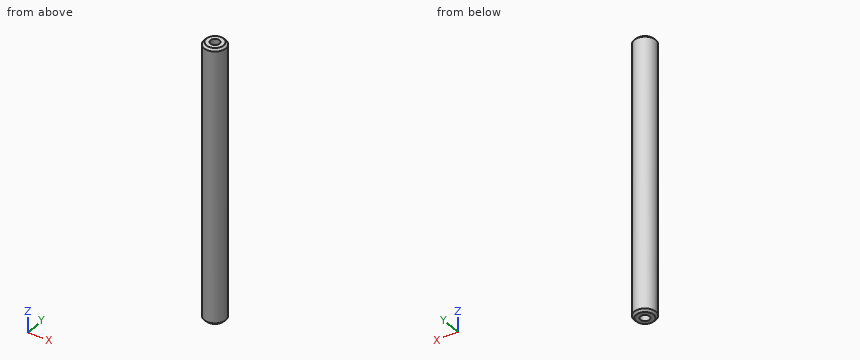
```python
from build123d import *

# Parameters (mm, degrees)
SKETCH3_R           = 3.96875
BOSS_EXTRUDE1_DEPTH = 50.8
CHAMFER1_SIZE       = 0.79375


with BuildPart() as part:
    # Sketch3 → Boss-Extrude1 (new body, symmetric)
    with BuildSketch(Plane.XY):
        Circle(SKETCH3_R)
    extrude(amount=BOSS_EXTRUDE1_DEPTH, both=True)

    # Chamfer1
    chamfer1_edges = [part.edges().sort_by_distance(p)[0] for p in [
        (-3.96875, 0, -50.8),
        (-3.96875, 0, 50.8),
    ]]
    chamfer(chamfer1_edges, length=CHAMFER1_SIZE)

    # Sketch6 → M4x0.7 Tapped Hole1 (revolve, cut)
    with BuildSketch(Plane(origin=(0, 0, -50.8), x_dir=(0, 1, 0), z_dir=(1, 0, 0))):
        Polygon((0, 0), (0, 15.991420021), (1.65, 15), (1.65, 0), align=None)
    m4x0_7_tapped_hole1 = revolve(axis=Axis((0, 0, -57.15), (0, 0, 1)), mode=Mode.SUBTRACT)

    # Mirror1: M4x0.7 Tapped Hole1 across plane
    add(m4x0_7_tapped_hole1.mirror(Plane.XY), mode=Mode.SUBTRACT)


solid = part.part
```
The model under review builds one solid part; all positions refer to its coordinate system, in mm. Round coordinates to 2 decimals unless told otherwise and drop trailing zeros. Order: outer loops, then holes, each group sorted by start corner. A loop starts at its lowest first (then second) coordinate and runs counter-clockwise, first axis right, second up. Notation, with made-up numbers: M 85,-26 L 123,-26 A22 ccw 123,-16 Z; hole C -30,53.5 d11. An arc over 180 degrees is marked long. Use a Markdown table: item, result.
1) Insertion check: pin 1 (2 mm diameter, centred on x = 1.5, z = -25, fed in from -Y); pin 2 (3 mm diameter, centred on x = 0, y = 0, fed in from -Z); pin 3 (1.5 mm diameter, centred on y = 3, z = 31.5, fed in from -X). Each pin has a flat end and moves straight along its axis. Give the tip position at first contact, or say it passes through.
Report:
| item | result |
|---|---|
| pin 1 | y = -3.94 |
| pin 2 | z = -35.71 |
| pin 3 | x = -3.27 |
2) Consider section A-A (z = 20.5). Write out the cut boundary in (x, y), then the cut area to 3 significant figures.
Report:
| item | result |
|---|---|
| outline | C 0,0 d7.94 |
| area | 49.5 mm^2 |
3) Wall thickness on line 1 along Y through (x, z) = (0, 43); line 2 along X through (y, z) = (-1.5, 36.5); line 3 along X through (y, z) = (-1.25, -45): over which ranges is each line inside the solid? List them lowest first. Write a range as [from, to].
Report:
| item | result |
|---|---|
| line 1 | [-3.97, -1.65], [1.65, 3.97] |
| line 2 | [-3.67, -0.69], [0.69, 3.67] |
| line 3 | [-3.77, -1.08], [1.08, 3.77] |
